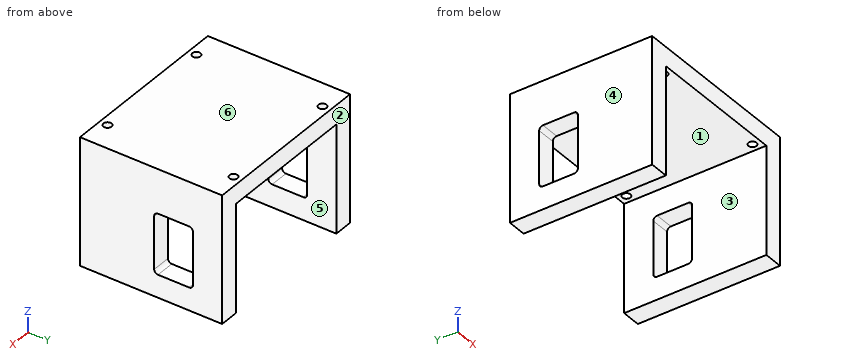
from build123d import *

# Parameters (mm, degrees)
ESQUISSE1_W               = 140
ESQUISSE1_H               = 112
BOSS_EXTRU_1_DEPTH        = 100
ESQUISSE2_W               = 110
ESQUISSE2_H               = 85
ENL_V_MAT_EXTRU_1_DEPTH   = 113
ESQUISSE3_W               = 47.5
ESQUISSE3_H               = 30.5
ENL_V_MAT_EXTRU_2_DEPTH   = 141
ESQUISSE4_R               = 3.175
ENL_V_MAT_EXTRU_3_DEPTH   = 16
SYM_TRIE2_COPY_1_SKETCH_R = 3.175
SYM_TRIE2_COPY_1_DEPTH    = 16
CONG_1_R                  = 3


with BuildPart() as part:
    # Esquisse1 → Boss.-Extru.1 (new body)
    with BuildSketch(Plane.XY):
        with Locations((-39.52963138, -51.586067687)):
            Rectangle(ESQUISSE1_W, ESQUISSE1_H)
    extrude(amount=BOSS_EXTRU_1_DEPTH)

    # Esquisse2 → Enlèv. mat.-Extru.1 (cut, through all)
    with BuildSketch(Plane(origin=(0, 4.413932313, 0), x_dir=(1, 0, 0), z_dir=(0, 1, 0))):
        with Locations((-39.52963138, -42.5)):
            Rectangle(ESQUISSE2_W, ESQUISSE2_H)
    extrude(amount=-ENL_V_MAT_EXTRU_1_DEPTH, mode=Mode.SUBTRACT)

    # Esquisse3 → Enlèv. mat.-Extru.2 (cut, through all)
    with BuildSketch(Plane.ZY.offset(109.52963138)):
        with Locations((41.617518417, -33.84820443)):
            Rectangle(ESQUISSE3_W, ESQUISSE3_H)
    extrude(amount=-ENL_V_MAT_EXTRU_2_DEPTH, mode=Mode.SUBTRACT)

    # Esquisse4 → Enlèv. mat.-Extru.3 (cut, through all)
    with BuildSketch(Plane(origin=(0, 0, 85), x_dir=(-1, 0, 0), z_dir=(0, 0, -1))):
        with Locations((-9.12036862, -1.936067687)):
            Circle(ESQUISSE4_R)
    enl_v_mat_extru_3 = extrude(amount=-ENL_V_MAT_EXTRU_3_DEPTH, mode=Mode.SUBTRACT)

    # Symétrie1: Enlèv. mat.-Extru.3 across plane
    add(enl_v_mat_extru_3.mirror(Plane(origin=(-39.52963138, 0, 0), x_dir=(0, 0, 1), z_dir=(1, 0, 0))), mode=Mode.SUBTRACT)

    # Symétrie2: Enlèv. mat.-Extru.3 across plane
    add(enl_v_mat_extru_3.mirror(Plane(origin=(0, -51.586067687, 0), x_dir=(0, 0, 1), z_dir=(0, -1, 0))), mode=Mode.SUBTRACT)

    # Symétrie2 copy 1 sketch → Symétrie2 copy 1 (cut, through all)
    with BuildSketch(Plane(origin=(-79.05926276, -103.172135375, 85), x_dir=(1, 0, 0), z_dir=(0, 0, -1))):
        with Locations((-9.12036862, -1.936067687)):
            Circle(SYM_TRIE2_COPY_1_SKETCH_R)
    extrude(amount=-SYM_TRIE2_COPY_1_DEPTH, mode=Mode.SUBTRACT)

    # Congé1
    cong_1_edges = [part.edges().sort_by_distance(p)[0] for p in [
        (-102.02963138, -49.09820443, 17.867518417),
        (-102.02963138, -18.59820443, 17.867518417),
        (-102.02963138, -18.59820443, 65.367518417),
        (-102.02963138, -49.09820443, 65.367518417),
        (22.97036862, -49.09820443, 17.867518417),
        (22.97036862, -18.59820443, 17.867518417),
        (22.97036862, -18.59820443, 65.367518417),
        (22.97036862, -49.09820443, 65.367518417),
    ]]
    fillet(cong_1_edges, radius=CONG_1_R)


solid = part.part
For this review, take the finished solid that the model builds, in its own axes (mm). Face numbers are marked on the shaded views. A direction names the side the tool comes from. Round coordinates to 2 decimals unless told otherwise and drop trailing zeros. Loops run counter-clockwise (first coordinate to the right, second up) from the corner with the lowest first, then second, coordinate; pieces in that order, holes last. Notation, with made-up numbers: (59.25, -3.5) - (90.25, -3.5) arc R9 ccw to (90.25, 13.5) - close; hole circle Ø8 at (15, -30.75). An arc over 180 degrees is marked (long way). Use one line per item in the form item = value.
1) We need section B-B on x = 20.5. Write out the cut boundary in (y, z).
Solutions:
outline = (-107.59, 0) - (4.41, 0) - (4.41, 100) - (-107.59, 100) - close; hole (-49.1, 20.87) arc R3 ccw to (-46.1, 17.87) - (-21.6, 17.87) arc R3 ccw to (-18.6, 20.87) - (-18.6, 62.37) arc R3 ccw to (-21.6, 65.37) - (-46.1, 65.37) arc R3 ccw to (-49.1, 62.37) - close
2) We need section D-D on y = -55. Write out the cut boundary in (x, z), then the cut area to 3 significant figures.
Solutions:
outline = (-109.53, 0) - (-94.53, 0) - (-94.53, 85) - (15.47, 85) - (15.47, 0) - (30.47, 0) - (30.47, 100) - (-109.53, 100) - close
area = 4,650 mm2
3) Wall thickness on probe 1 along Y at (x, z) = (12, 89); probe 2 along X at (y, z) = (-6, 6); probe 3 along Z at (x, y) = (-27, -42): over which ranges is each line inside the solid? List them lowest first.
Solutions:
probe_1 = -107.59 to -102.57, -99.9 to -3.27, -0.6 to 4.41
probe_2 = -109.53 to -94.53, 15.47 to 30.47
probe_3 = 85 to 100
4) We need section C-C on z = 74. Write out the cut boundary in (x, y).
Solutions:
outline = (-109.53, -107.59) - (-94.53, -107.59) - (-94.53, 4.41) - (-109.53, 4.41) - close; (15.47, -107.59) - (30.47, -107.59) - (30.47, 4.41) - (15.47, 4.41) - close
5) Tool access review of the marked faces 5 and 6: name each direction out of +Z, -Z, +X, -X, +Y, -Y from which nothing blocks a thin tool from reaching the whole face with its end or side.
Solutions:
face_5 = -Z, +Y, -Y
face_6 = +Z, +X, -X, +Y, -Y
6) Mouldability with a two-part tool opening along X and no side actions: class the marked faces 1, 2, 3 and 4 as pulls with the +X half, pulls with the -X half, needs draft (parallel to the pull), parting line crosses it, or undercut.
Solutions:
face_1 = undercut
face_2 = needs draft
face_3 = undercut
face_4 = pulls with the -X half
7) Clearance check with a flat-ended pin moving along its axis: P1, Ø2, axis at x = -2.5, y = -84, coming from the -Z side. State where the tip first meets the part, or that it passes through.
Solutions:
P1 = 85
8) We need section A-A on z = 34. Write out the cut boundary in (x, y), then the cut area to 4 significant figures.
Solutions:
outline = (-109.53, -107.59) - (-94.53, -107.59) - (-94.53, -49.1) - (-109.53, -49.1) - close; (-109.53, -18.6) - (-94.53, -18.6) - (-94.53, 4.41) - (-109.53, 4.41) - close; (15.47, -107.59) - (30.47, -107.59) - (30.47, -49.1) - (15.47, -49.1) - close; (15.47, -18.6) - (30.47, -18.6) - (30.47, 4.41) - (15.47, 4.41) - close
area = 2,445 mm2
